Model file for the job. Use its own axes, mm. Face numbers are marked on the shaded views. Round coordinates to 2 decimals unless told otherwise and drop trailing zeros. Write each loop counter-clockwise with the first axis right and the second up, starting at its lowest first coordinate (ties: lowest second). Pieces come first, ordered by that corner, then holes.
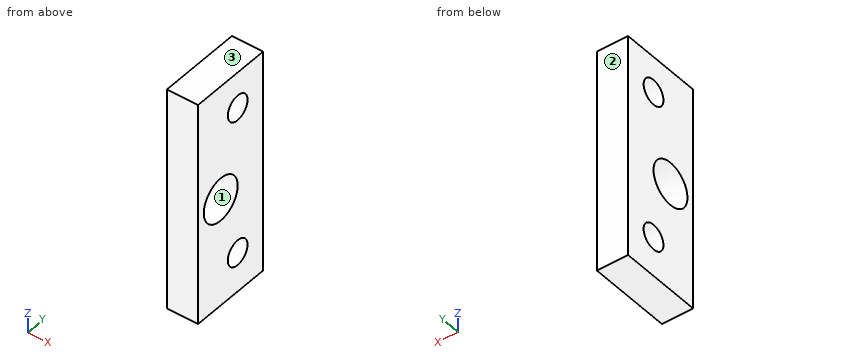
Autodesk Inventor part; units mm, degrees
ref_plane "YZ Plane" through (0, 0, 0) normal (1, 0, 0) x (0, 1, 0)
ref_plane "XZ Plane" through (0, 0, 0) normal (0, 1, 0) x (-1, 0, 0)
ref_plane "XY Plane" through (0, 0, 0) normal (0, 0, 1) x (1, 0, 0)
sketch "Sketch1" plane through (0, 0, 0) normal (1, 0, 0) x (0, 1, 0)
  line L0 (0, 0) -> (11.5, 0)
  line L1 (11.5, 0) -> (11.5, 31)
  line L2 (11.5, 31) -> (0, 31)
  line L3 (0, 31) -> (0, 0)
  line L4 (0, 15) -> (4, 15) construction
  circle A0 centre (4, 15) radius 3
  line L5 (7, 26) -> (7, 5.5) construction
  circle A1 centre (7, 26) radius 1.75
  circle A2 centre (7, 5.5) radius 1.75
  dimension "d0" = 4
  dimension "d1" = 6
  dimension "d2" = 20.5
  dimension "d3" = 9.5
  dimension "d4" = 3.5
  dimension "d5" = 7
  dimension "d6" = 11.5
  dimension "d7" = 15
  dimension "d8" = 16
extrude "Extrusion1" add sketch "Sketch1" along normal blind 4.3
properties part number "TrayPanelL"
1) Pull direction Z, two halves, no side cores. Call the marked faces 1, 2 and 3: released by +Z, released by -Z, zero draft, split by the parting line, or undercut.
2) Flat gauge pin, fed straight in: pin 1 Ø3 at (y, z) = (7, 26) entering from +X. Where does the tip first touch, or does it go through?
3) Cut at A-A on z = 26. List the corners of the cut face in (x, y), and give its area (3 significant figures).
4) Cut at D-D on y = 6.5. List the corners of the cut face in (x, z), and give its area (3 significant figures).
5) Cut at C-C on y = 4. List the corners of the cut face in (x, z), and give its area (4 significant figures).
6) Wall check: probe 1 along Z at (x, y) = (2.3, 4); probe 2 along Z at (x, y) = (1.05, 8); probe 3 along Y at (x, z) = (4.15, 14.5). Give the ranges that are in metal, low to high.
7) Cut at B-B on x = 3.8. List the corners of the cut face in (y, z), and give its area (3 significant figures).
Result sheet:
1. face 1: undercut
1. face 2: zero draft
1. face 3: released by +Z
2. pin 1: passes through
3. outline: (0, 0) - (4.3, 0) - (4.3, 5.25) - (0, 5.25) - close; (0, 8.75) - (4.3, 8.75) - (4.3, 11.5) - (0, 11.5) - close
3. area: 34.4 mm2
4. outline: (0, 0) - (4.3, 0) - (4.3, 3.82) - (0, 3.82) - close; (0, 7.18) - (4.3, 7.18) - (4.3, 13.34) - (0, 13.34) - close; (0, 16.66) - (4.3, 16.66) - (4.3, 24.32) - (0, 24.32) - close; (0, 27.68) - (4.3, 27.68) - (4.3, 31) - (0, 31) - close
4. area: 90.2 mm2
5. outline: (0, 0) - (4.3, 0) - (4.3, 12) - (0, 12) - close; (0, 18) - (4.3, 18) - (4.3, 31) - (0, 31) - close
5. area: 107.5 mm2
6. probe 1: z = 0 to 12, 18 to 31
6. probe 2: z = 0 to 4.06, 6.94 to 24.56, 27.44 to 31
6. probe 3: y = 0 to 1.04, 6.96 to 11.5
7. outline: (0, 0) - (11.5, 0) - (11.5, 31) - (0, 31) - close; hole circle Ø6 at (4, 15); hole circle Ø3.5 at (7, 5.5); hole circle Ø3.5 at (7, 26)
7. area: 309 mm2
